from build123d import *

# Parameters (mm, degrees)
BOSS_EXTRUDE1_DEPTH      = 44.45
BOSS_EXTRUDE1_DEPTH_BACK = 63.5
SKETCH1_W                = 431.8
SKETCH1_H                = 431.8
CUT_EXTRUDE1_DEPTH       = 324.85
CUT_EXTRUDE1_DEPTH_BACK  = 324.85
SKETCH2_OUTSIDE_W        = 557.826
SKETCH2_OUTSIDE_H        = 557.826
CUT_EXTRUDE5_DEPTH       = 22.225
SHELL1_T                 = -19.05
CUT_EXTRUDE3_DEPTH       = 3.175
SKETCH5_W                = 120.0338561
SKETCH5_H                = 81.699458139
CUT_EXTRUDE4_DEPTH       = 393.7


with BuildPart() as part:
    # Sketch1 → Boss-Extrude1 (new, two sides: drawn at the far end of the back side and taken through both)
    with BuildSketch(Plane.XY.offset(-BOSS_EXTRUDE1_DEPTH_BACK)):
        Rectangle(SKETCH1_W, SKETCH1_H)
    extrude(amount=BOSS_EXTRUDE1_DEPTH + BOSS_EXTRUDE1_DEPTH_BACK)

    # Sketch2 outside → Cut-Extrude1 (cut, two sides: drawn at the far end of the back side and taken through both)
    with BuildSketch(Plane.XY.offset(44.45).offset(-CUT_EXTRUDE1_DEPTH_BACK)):
        Rectangle(SKETCH2_OUTSIDE_W, SKETCH2_OUTSIDE_H)
        Polygon((-215.9, 89.428708116), (-215.9, -89.428708116), (-89.428708116, -215.9), (89.428708116, -215.9), (215.9, -89.428708116), (215.9, 89.428708116), (89.428708116, 215.9), (-89.428708116, 215.9), align=None, mode=Mode.SUBTRACT)
    extrude(amount=CUT_EXTRUDE1_DEPTH + CUT_EXTRUDE1_DEPTH_BACK, mode=Mode.SUBTRACT)

    # Sketch6 → Cut-Extrude5 (cut, symmetric)
    with BuildSketch(Plane(origin=(0, 0, 0), x_dir=(0, 0, -1), z_dir=(1, 0, 0))):
        Polygon((-12.7, 215.9), (-3.175, -215.9), (63.5, -215.9), (63.5, 215.9), align=None)
    extrude(amount=CUT_EXTRUDE5_DEPTH, both=True, mode=Mode.SUBTRACT)

    # Shell1
    shell1_openings = [part.faces().sort_by_distance(p)[0] for p in [
        (0, 0, 44.45),
    ]]
    offset(amount=SHELL1_T, openings=shell1_openings, kind=Kind.INTERSECTION)

    # Sketch4 → Cut-Extrude3 (cut)
    with BuildSketch(Plane.XY.offset(44.45)):
        Polygon((85.483323935, 206.375), (-85.483323935, 206.375), (-206.375, 85.483323935), (-206.375, -85.483323935), (-85.483323935, -206.375), (85.483323935, -206.375), (206.375, -85.483323935), (206.375, 85.483323935), align=None)
    extrude(amount=-CUT_EXTRUDE3_DEPTH, mode=Mode.SUBTRACT)

    # Sketch5 → Cut-Extrude4 (cut)
    with BuildSketch(Plane(origin=(0, -196.85, 0), x_dir=(1, 0, 0), z_dir=(0, 1, 0))):
        with Locations((1.389541827, 3.60027093)):
            Rectangle(SKETCH5_W, SKETCH5_H)
    extrude(amount=CUT_EXTRUDE4_DEPTH, mode=Mode.SUBTRACT)


solid = part.part
Can you work these out from the model? Positions are in its coordinate system, mm. A direction names the side the tool comes from. Give positions to 0.01 mm unless a question says otherwise; leave off trailing zeros. Loops run counter-clockwise (first coordinate to the right, second up) from the corner with the lowest first, then second, coordinate; pieces in that order, holes last. Notation, with made-up numbers: (87.5, 39) -> (126.5, 39) arc R24 ccw to (126.5, 56) -> close; hole circle Ø9 at (10, 40). An arc over 180 degrees is marked (long way). Use one line per item in the form item = value.
1) If we section it at D-D (x = -73.5): Please give me the cut outline in (y, z) (3 decimals), plus the area to 3 significant figures.
Answers:
outline = (-215.9, -63.5) -> (215.9, -63.5) -> (215.9, 44.45) -> (206.375, 44.45) -> (206.375, 41.275) -> (196.85, 41.275) -> (196.85, -44.45) -> (-196.85, -44.45) -> (-196.85, 41.275) -> (-206.375, 41.275) -> (-206.375, 44.45) -> (-215.9, 44.45) -> close
area = 11,600 mm²
2) Will these pins go through, and if not, where does the flat tip stop? pin 1 (1.5 mm diameter, centred on x = -97, y = 34.5, fed in from +Z); pin 2 (5 mm diameter, centred on y = 109, z = 14, fed in from -X).
Answers:
pin_1 = -44.45
pin_2 = -198.83
3) If we section it at A-A (z = -51): Please give me the cut outline in (x, y) (3 decimals), plus the area to 3 significant figures.
Answers:
outline = (-215.9, -89.429) -> (-89.429, -215.9) -> (-22.225, -215.9) -> (-22.225, 215.9) -> (-89.429, 215.9) -> (-215.9, 89.429) -> close; (22.225, -215.9) -> (89.429, -215.9) -> (215.9, -89.429) -> (215.9, 89.429) -> (89.429, 215.9) -> (22.225, 215.9) -> close
area = 135,000 mm²
4) For faces 5 (the face through (151.78, -153.55, -10.28)), 6 (the face through (-146.78, -145.08, 42.88)), which set-ups out of +Z, -Z, +X, -X, +Y, -Y let a thin tool reach every point of the face, with its end or its side?
Answers:
face_5 = +Z, -Z, +X, -Y
face_6 = +Z
5) I need wall thicknesses on line 1 along X through (y, z) = (-12, 9.5). Which ranges of the line are inside material? Lowest first, please.
Answers:
line_1 = -215.9 to -196.85, 196.85 to 215.9
6) We'd pull the mould along X, two halves only. Please class faces 1 (the face through (-1, -196.85, 7)), 2 (the face through (-1, -215.9, 14)), 3 (the face through (215.9, -1, -10)), 4 (the face through (-196.85, -1, -2)): released by +X, released by -X, zero draft, split by the parting line, or undercut.
Answers:
face_1 = undercut
face_2 = zero draft
face_3 = released by +X
face_4 = undercut
7) If we section it at C-C (y = -72.5): Please give me the cut outline in (x, z) (3 decimals).
Answers:
outline = (-215.9, -63.5) -> (-22.225, -63.5) -> (-22.225, -44.45) -> (-196.85, -44.45) -> (-196.85, 41.275) -> (-206.375, 41.275) -> (-206.375, 44.45) -> (-215.9, 44.45) -> close; (22.225, -63.5) -> (215.9, -63.5) -> (215.9, 44.45) -> (206.375, 44.45) -> (206.375, 41.275) -> (196.85, 41.275) -> (196.85, -44.45) -> (22.225, -44.45) -> close
8) If we section it at B-B (x = -12.5): Please give me the cut outline in (y, z) (3 decimals), plus the area to 3 significant figures.
Answers:
outline = (-215.9, 3.175) -> (-196.85, 3.595) -> (-196.85, 41.275) -> (-206.375, 41.275) -> (-206.375, 44.45) -> (-215.9, 44.45) -> close; (196.85, 12.28) -> (215.9, 12.7) -> (215.9, 44.45) -> (206.375, 44.45) -> (206.375, 41.275) -> (196.85, 41.275) -> close
area = 1,330 mm²
